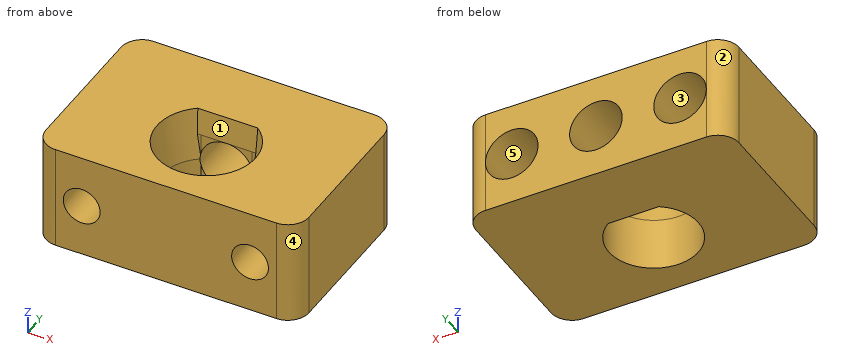
Autodesk Inventor part; units mm, degrees
ref_plane "YZ Plane" through (0, 0, 0) normal (1, 0, 0) x (0, 1, 0)
ref_plane "XZ Plane" through (0, 0, 0) normal (0, 1, 0) x (-1, 0, 0)
ref_plane "XY Plane" through (0, 0, 0) normal (0, 0, 1) x (1, 0, 0)
sketch "Sketch1" plane through (0, 0, 0) normal (0, 0, 1) x (1, 0, 0)
  circle A0 centre (0, 0) radius 4.25
  line L0 (-2.4109, 3.5) -> (2.4109, 3.5)
  line L1 (-12.5, 10) -> (12.5, 10)
  line L2 (12.5, 10) -> (12.5, -7)
  line L3 (12.5, -7) -> (-12.5, -7)
  line L4 (-12.5, -7) -> (-12.5, 10)
  dimension "d0" = 8.5
  dimension "d1" = 3.5
  dimension "d2" = 25
  dimension "d3" = 12.5
  dimension "d4" = 17
  dimension "d5" = 10
extrude "Extrusion1" add sketch "Sketch1" along normal blind 10 contours L0 A0 | L1 L2 L3 L4 picked at (-0.1705, 3.7397)
sketch "Sketch2" plane through (-12.5, 10, 0) normal (0, 1, 0) x (1, 0, 0)
  line L0 (25, -10) -> (0, -10)
  line L1 (25, 0) -> (0, 0)
  line L2 (0, 0) -> (0, -10)
  point P0 (12.5, 0)
  point P1 (4.5, -5)
  dimension "d8" = 10
  dimension "d9" = 5
  dimension "d18" = 8
hole "Hole1" at (-8, 10, 5) direction (0, -1, 0) diameter 3.5 depth 17 counterbore diameter 5 counterbore depth 5
mirror "Mirror1" about plane through (0, 0, 0) normal (1, 0, 0) of "Hole1"
sketch "Sketch3" plane through (-12.5, 10, 0) normal (0, 1, 0) x (1, 0, 0)
  line L0 (25, -10) -> (0, -10)
  line L1 (25, 0) -> (0, 0)
  line L2 (25, 0) -> (25, -10)
  line L3 (0, 0) -> (0, -10)
  point P0 (12.5, 0)
  point P1 (12.5, -5)
  dimension "d19" = 10
  dimension "d20" = 5
  dimension "d21" = 25
  dimension "d22" = 12.5
hole "Hole2" at (0, 10, 5) direction (0, -1, 0) diameter 5 end up to surface
fillet "Fillet1" radius 2 4 edges at (-12.5, 10, 5) (12.5, 10, 5) (12.5, -7, 5) (-12.5, -7, 5)
chamfer "Chamfer1" distance 5 angle 5 1 edges at (0, -4.25, 10)
chamfer "Chamfer2" distance 2.5 angle 5 1 edges at (0, 3.5, 10) measured on face at (0, 3.5, 9.1667)
properties part number "pendulum_adapter" material "ABS Plastic"
The listing builds one solid part. Answer for the finished solid, in the listing's coordinates (mm). Face numbers are marked on the shaded views. A direction names the side the tool comes from. Coordinates: 2 decimals unless noted, no trailing zeros. Write each loop counter-clockwise with the first axis right and the second up, starting at its lowest first coordinate (ties: lowest second). Pieces come first, ordered by that corner, then holes. Notation, with made-up numbers: (-25.5, 64.25) -> (-17.5, 64.25) arc R30 ccw to (-17.5, 91.25) -> close; hole circle Ø7 at (-24, 31). An arc over 180 degrees is marked (long way). One line per question, with ' | ' between items.
1. Given pin 1 Ø1 at (x, y) = (-3.5, 1) entering from -Z (3 decimals), flat-ended and moving along its own axis, determine where the tip first touches the part or whether it passes through.
Verdict:
pin 1: passes through
2. Which of the six approach directions +Z, -Z, +X, -X, +Y, -Y give full straight-line access (tool end or side, diameter ignored) to the marked faces 4 and 5?
Verdict:
face 4: +Z, -Z, +X, -Y | face 5: +Y
3. For a pull along Y with two mould halves and no side action, classify the marked faces 1, 2 and 3 as released by +Y, released by -Y, zero draft, split by the parting line, or undercut.
Verdict:
face 1: undercut | face 2: released by +Y | face 3: zero draft
4. Straight lines are drawn through the part: line 1 (X direction, y = 6.1, z = 5); line 2 (X direction, y = 0, z = 1.2); line 3 (X direction, y = -0.5, z = 5). For each, find the intervals that lie inside material, in ascending order.
Verdict:
line 1: x = -12.5 to -10.5, -5.5 to -2.5, 2.5 to 5.5, 10.5 to 12.5 | line 2: x = -12.5 to -4.25, 4.25 to 12.5 | line 3: x = -12.5 to -9.75, -6.25 to -4.22, 4.22 to 6.25, 9.75 to 12.5
5. Section C-C (y = 5.75) is taken. Determine the outline of the cut face in (x, z).
Verdict:
outline: (-12.5, 0) -> (12.5, 0) -> (12.5, 10) -> (-12.5, 10) -> close; hole circle Ø5 at (-8, 5); hole circle Ø5 at (0, 5); hole circle Ø5 at (8, 5)
6. Section B-B (y = 0) is taken. Determine the outline of the cut face in (x, z), and give its area (3 significant figures).
Verdict:
outline: (-12.5, 0) -> (-4.25, 0) -> (-4.25, 5) -> (-4.69, 10) -> (-12.5, 10) -> close; (4.25, 0) -> (12.5, 0) -> (12.5, 10) -> (4.69, 10) -> (4.25, 5) -> close; hole circle Ø3.5 at (-8, 5); hole circle Ø3.5 at (8, 5) | area: 144 mm^2
7. Section A-A (x = -8) is taken. Determine the outline of the cut face in (y, z).
Verdict:
outline: (-7, 0) -> (10, 0) -> (10, 2.5) -> (5, 2.5) -> (5, 3.25) -> (-7, 3.25) -> close; (-7, 6.75) -> (5, 6.75) -> (5, 7.5) -> (10, 7.5) -> (10, 10) -> (-7, 10) -> close
8. Section D-D (z = 1.5) is taken. Determine the outline of the cut face in (x, y), and give its area (3 significant figures).
Verdict:
outline: (-12.5, -5) arc R2 ccw to (-10.5, -7) -> (10.5, -7) arc R2 ccw to (12.5, -5) -> (12.5, 8) arc R2 ccw to (10.5, 10) -> (-10.5, 10) arc R2 ccw to (-12.5, 8) -> close; hole (-2.41, 3.5) arc R4.25 ccw (long way) to (2.41, 3.5) -> close | area: 367 mm^2
